Part model, mm, in its own coordinate system. Face numbers are marked on the shaded views. A direction names the side the tool comes from. Coordinates: 2 decimals unless noted, no trailing zeros. Loops run counter-clockwise (first coordinate to the right, second up) from the corner with the lowest first, then second, coordinate; pieces in that order, holes last. Notation, with made-up numbers: (22, 72) - (54, 72) arc R18 cw to (54, 98) - close; hole circle Ø10 at (-7, 38.25). An arc over 180 degrees is marked (long way). Answer as CSV lines item,"result".
from build123d import *

# Parameters (mm, degrees)
SKETCH1_W                                       = 25
SKETCH1_H                                       = 34
BOSS_EXTRUDE1_DEPTH                             = 20
SKETCH2_W                                       = 30
SKETCH2_H                                       = 53.5
BOSS_EXTRUDE2_DEPTH                             = 3
FILLET1_R                                       = 5
SKETCH3_W                                       = 22.5
SKETCH3_H                                       = 30.5
CUT_EXTRUDE1_DEPTH                              = 22
FILLET2_R                                       = 3
SKETCH4_W                                       = 2
SKETCH4_H                                       = 6
SKETCH4_H_2                                     = 5
BOSS_EXTRUDE3_DEPTH                             = 20
CHAMFER1_SIZE                                   = 0.5
CSK_FOR_M3_FLAT_HEAD_MACHINE_SCREW1_D           = 3.4
CSK_FOR_M3_FLAT_HEAD_MACHINE_SCREW1_DEPTH       = 3
CSK_FOR_M3_FLAT_HEAD_MACHINE_SCREW1_CSINK_D     = 6.3
CSK_FOR_M3_FLAT_HEAD_MACHINE_SCREW1_CSINK_ANGLE = 90
CSK_FOR_M3_FLAT_HEAD_MACHINE_SCREW1_TIP         = 1.021463052


with BuildPart() as part:
    # Sketch1 → Boss-Extrude1 (new body)
    with BuildSketch(Plane(origin=(0, 0, 0), x_dir=(1, 0, 0), z_dir=(0, 1, 0))):
        Rectangle(SKETCH1_W, SKETCH1_H)
    extrude(amount=-BOSS_EXTRUDE1_DEPTH)

    # Sketch2 → Boss-Extrude2 (add)
    with BuildSketch(Plane(origin=(0, 0, 0), x_dir=(1, 0, 0), z_dir=(0, 1, 0))):
        Rectangle(SKETCH2_W, SKETCH2_H)
    extrude(amount=BOSS_EXTRUDE2_DEPTH)

    # Fillet1
    fillet1_edges = [part.edges().sort_by_distance(p)[0] for p in [
        (15, 1.5, 26.75),
        (15, 1.5, -26.75),
        (-15, 1.5, -26.75),
        (-15, 1.5, 26.75),
    ]]
    fillet(fillet1_edges, radius=FILLET1_R)

    # Sketch3 → Cut-Extrude1 (cut)
    with BuildSketch(Plane(origin=(0, 3, 0), x_dir=(1, 0, 0), z_dir=(0, 1, 0))):
        Rectangle(SKETCH3_W, SKETCH3_H)
    extrude(amount=-CUT_EXTRUDE1_DEPTH, mode=Mode.SUBTRACT)

    # Fillet2
    fillet2_edges = [part.edges().sort_by_distance(p)[0] for p in [
        (11.25, -8, -15.25),
        (11.25, -8, 15.25),
        (-11.25, -8, 15.25),
        (-11.25, -8, -15.25),
    ]]
    fillet(fillet2_edges, radius=FILLET2_R)

    # Sketch4 → Boss-Extrude3 (add)
    with BuildSketch(Plane(origin=(0, -19, 0), x_dir=(1, 0, 0), z_dir=(0, 1, 0))):
        with Locations((4, 0)):
            Rectangle(SKETCH4_W, SKETCH4_H)
        with Locations((-4, 6.5)):
            Rectangle(SKETCH4_W, SKETCH4_H_2)
        with Locations((-4, -6.5)):
            Rectangle(SKETCH4_W, SKETCH4_H_2)
    extrude(amount=BOSS_EXTRUDE3_DEPTH)

    # Chamfer1
    chamfer1_edges = [part.edges().sort_by_distance(p)[0] for p in [
        (-3, 1, -6.5),
        (-4, 1, -9),
        (-5, 1, -6.5),
        (-4, 1, -4),
        (-5, 1, 6.5),
        (-4, 1, 9),
        (-3, 1, 6.5),
        (-4, 1, 4),
        (5, 1, 0),
        (4, 1, -3),
        (3, 1, 0),
        (4, 1, 3),
    ]]
    chamfer(chamfer1_edges, length=CHAMFER1_SIZE)

    # CSK for M3 Flat Head Machine Screw1
    with Locations(Plane(origin=(0, 3, -21.5), x_dir=(0, 0, 1), z_dir=(0, 1, 0))):
        with Locations((0, 0), (43, 0)):
            CounterSinkHole(CSK_FOR_M3_FLAT_HEAD_MACHINE_SCREW1_D / 2, CSK_FOR_M3_FLAT_HEAD_MACHINE_SCREW1_CSINK_D / 2, depth=CSK_FOR_M3_FLAT_HEAD_MACHINE_SCREW1_DEPTH, counter_sink_angle=CSK_FOR_M3_FLAT_HEAD_MACHINE_SCREW1_CSINK_ANGLE)
            with Locations((0, 0, -(CSK_FOR_M3_FLAT_HEAD_MACHINE_SCREW1_DEPTH + CSK_FOR_M3_FLAT_HEAD_MACHINE_SCREW1_TIP / 2))):  # 118° drill point
                Cone(0, CSK_FOR_M3_FLAT_HEAD_MACHINE_SCREW1_D / 2, CSK_FOR_M3_FLAT_HEAD_MACHINE_SCREW1_TIP, mode=Mode.SUBTRACT)


solid = part.part
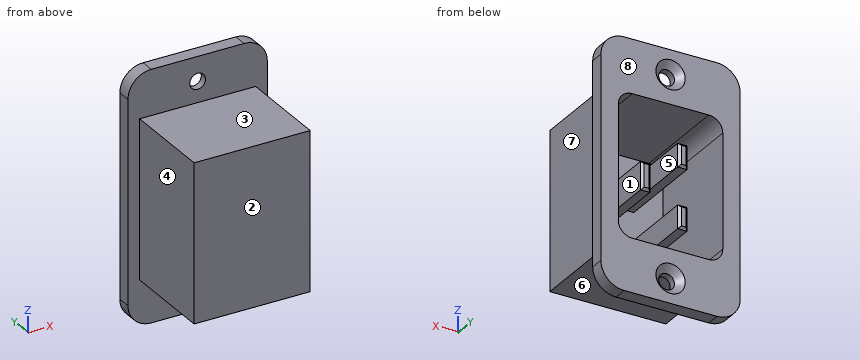
Q1. Wall check: L1, parallel to Z at x = 0, y = 0.35; L2, parallel to Z at x = -3.5, y = -1.5; L3, parallel to X at y = -12.25, z = 1.5. Give the ranges that are in metal, low to high.
Results:
L1,"z = -26.75 to -23.2, -19.8 to -15.25, 15.25 to 19.8, 23.2 to 26.75"
L2,"z = -17 to -15.25, -9 to -4, 4 to 9, 15.25 to 17"
L3,"x = -12.5 to -11.25, 3 to 5, 11.25 to 12.5"
Q2. Saw through at C-C (z = -10.5). Give the cut face in (x, y).
Results:
outline,"(-15, 0) - (-12.5, 0) - (-12.5, -20) - (12.5, -20) - (12.5, 0) - (15, 0) - (15, 3) - (11.25, 3) - (11.25, -19) - (-11.25, -19) - (-11.25, 3) - (-15, 3) - close"
Q3. Saw through at D-D (x = -7.5). Give the cut face in (y, z), then the cut area to 4 significant figures.
Results:
outline,"(-20, -17) - (0, -17) - (0, -26.75) - (3, -26.75) - (3, -15.25) - (-19, -15.25) - (-19, 15.25) - (3, 15.25) - (3, 26.75) - (0, 26.75) - (0, 17) - (-20, 17) - close"
area,"169.5 mm^2"
Q4. Which spindle directions (+Z, -Z, +X, -X, +Y, -Y) get a long thin tool onto all of the face, cutting with end or side? Do the marked faces 4, 5, 6, 7 and 8. Say none if no direction does.
Results:
face 4,"+Z, -Z, -X, -Y"
face 5,"+Y"
face 6,"-Z, +X, -X, -Y"
face 7,"+Z, -Z, +X, -Y"
face 8,"+Z, -Z, +X, -X, +Y"
Q5. Saw through at A-A (y = -5.25). Give the cut face in (x, z), then the cut area to 3 significant figures.
Results:
outline,"(-12.5, -17) - (12.5, -17) - (12.5, 17) - (-12.5, 17) - close; (-5, -9) - (-3, -9) - (-3, -4) - (-5, -4) - close; (-5, 4) - (-3, 4) - (-3, 9) - (-5, 9) - close; (3, -3) - (5, -3) - (5, 3) - (3, 3) - close; hole (-11.25, -12.25) arc R3 ccw to (-8.25, -15.25) - (8.25, -15.25) arc R3 ccw to (11.25, -12.25) - (11.25, 12.25) arc R3 ccw to (8.25, 15.25) - (-8.25, 15.25) arc R3 ccw to (-11.25, 12.25) - close"
area,"203 mm^2"
Q6. Flat gauge pins, fed straight in: pin 1 (6 mm diameter, centred on y = -14, z = -3.5, fed in from -X); pin 2 (4 mm diameter, centred on x = -8.5, y = -12, fed in from +Z); pin 3 (0.5 mm diameter, centred on x = 4, z = -0.5, fed in from +Y); pin 4 (5 mm diameter, centred on y = -12.5, z = 21, fed in from +X). Where does each tip first touch, or does it go through?
Results:
pin 1,"stops at x = -12.5"
pin 2,"stops at z = 17"
pin 3,"stops at y = 1"
pin 4,"passes through"
Q7. Saw through at B-B (x = 0). Give the cut face in (y, z).
Results:
outline,"(-20, -17) - (0, -17) - (0, -19.8) - (1.55, -19.8) - (3, -18.35) - (3, -15.25) - (-19, -15.25) - (-19, 15.25) - (3, 15.25) - (3, 18.35) - (1.55, 19.8) - (0, 19.8) - (0, 17) - (-20, 17) - close; (0, -26.75) - (3, -26.75) - (3, -24.65) - (1.55, -23.2) - (0, -23.2) - close; (0, 23.2) - (1.55, 23.2) - (3, 24.65) - (3, 26.75) - (0, 26.75) - close"
Q8. Two-plate mould, pull along Z, no slides. Class the marked faces 1, 2 and 3: released by +Z, released by -Z, zero draft, split by the parting line, or undercut.
Results:
face 1,"undercut"
face 2,"zero draft"
face 3,"released by +Z"
